Part model, mm, in its own coordinate system. A direction names the side the tool comes from. Coordinates: 2 decimals unless noted, no trailing zeros. Order: outer loops, then holes, each group sorted by start corner. A loop starts at its lowest first (then second) coordinate and runs counter-clockwise, first axis right, second up.
from build123d import *

# Parameters (mm, degrees)
F1_DEPTH = 12.7
F4_SIZE  = 6.35
F3_R     = 3.81
F5_DEPTH = 58.372665
F6_R     = 8.89
F7_DEPTH = 12.7
F8_SIZE  = 5.08


with BuildPart() as f1:
    # F0 (on Top) → F1 (new body, symmetric)
    with BuildSketch(Plane.XY):
        Polygon((-31.75, 9.525), (-31.75, 0), (-12.7, 0), (-12.7, -1.905), (-1.905, -12.7), (0, -12.7), (0, -31.75), (9.525, -31.75), (9.525, 9.525), align=None)
    extrude(amount=F1_DEPTH, both=True)

    # F4
    f4_edges = [f1.edges().sort_by_distance(p)[0] for p in [
        (9.525, 9.525, 0),
    ]]
    chamfer(f4_edges, length=F4_SIZE)

    # F3 (on face) → F5 (cut, through all)
    with BuildSketch(Plane(origin=(9.525, 9.525, 0), x_dir=(0.707107, -0.707107, 0), z_dir=(-0.707107, -0.707107, 0))):
        Circle(F3_R)
    extrude(amount=F5_DEPTH, mode=Mode.SUBTRACT)

    # F6 (on face) → F7 (cut)
    with BuildSketch(Plane(origin=(9.525, 9.525, 0), x_dir=(0.707107, -0.707107, 0), z_dir=(-0.707107, -0.707107, 0))):
        Circle(F6_R)
    extrude(amount=F7_DEPTH, mode=Mode.SUBTRACT)

    # F8
    f8_edges = [f1.edges().sort_by_distance(p)[0] for p in [
        (9.525, -31.75, 0),
        (-31.75, 9.525, 0),
    ]]
    chamfer(f8_edges, length=F8_SIZE)


solid = f1.part
Q1. Cut at B-B on y = -22. Write the cut outline in (x, z) (3 decimals).
Results list:
outline: (0, -12.7) - (9.525, -12.7) - (9.525, 12.7) - (0, 12.7) - close
Q2. Cut at C-C on z = -7. Write the cut outline in (x, y) (3 decimals).
Results list:
outline: (-31.75, 0) - (-12.7, 0) - (-12.7, -1.905) - (-1.905, -12.7) - (0, -12.7) - (0, -31.75) - (4.445, -31.75) - (9.525, -26.67) - (9.525, 1.775) - (4.42, -3.33) - (-3.33, 4.42) - (1.775, 9.525) - (-26.67, 9.525) - (-31.75, 4.445) - close
Q3. Mould opens along X. For faces 1 (the face through (9.525, -12, 0)), 2 (the face through (-31.75, 2, 0)), 3 (the face through (8.84, -3.15, 2.67)) say: pulls with the +X half, pulls with the -X half, needs draft (parallel to the pull), parting line crosses it, or undercut.
Results list:
face 1: pulls with the +X half
face 2: pulls with the -X half
face 3: undercut
Q4. Wall check: line 1 along Y through (x, z) = (-26, 10.5) (3 decimals); line 2 along Z through (x, y) = (1.5, 0); line 3 along Z through (x, y) = (6, 5.5). Give the ranges that are in metal, low to high.
Results list:
line 1: y = 0 to 9.525
line 2: z = -12.7 to -8.83, 8.83 to 12.7
line 3: z = -12.7 to -8.88, 8.88 to 12.7
Q5. Pin check, flat tips, straight feed: pin 1 Ø0.6 at (y, z) = (-1, 0.5) entering from -X; pin 2 Ø4 at (x, z) = (-17.5, -9.5) entering from -Y; pin 3 Ø15 at (y, z) = (-24, -5) entering from -X. Stop position of each tip, or through.
Results list:
pin 1: stops at x = -12.7
pin 2: stops at y = 0
pin 3: stops at x = 0
Q6. Which spindle directions (+Z, -Z, +X, -X, +Y, -Y) get a long thin tool onto all of the face, cutting with end or side? Do faces 4 (the face through (3.25, -2.16, -1.85)), 5 (the face through (-2, -6, -12.7)), 6 (the face through (0, -22, 0)). Say none if no direction does.
Results list:
face 4: none
face 5: -Z, +X, -X, +Y, -Y
face 6: +Z, -Z, -X, -Y
Q7. Cut at A-A on z = 3. Write the cut outline in (x, y) (3 decimals).
Results list:
outline: (-31.75, 0) - (-12.7, 0) - (-12.7, -1.905) - (-8.963, -5.642) - (-1.116, 2.205) - (-5.373, 6.462) - (-2.31, 9.525) - (-26.67, 9.525) - (-31.75, 4.445) - close; (-5.642, -8.963) - (-1.905, -12.7) - (0, -12.7) - (0, -31.75) - (4.445, -31.75) - (9.525, -26.67) - (9.525, -2.31) - (6.462, -5.373) - (2.205, -1.116) - close
